Verification items for the finished model (mm, model axes). Face numbers are marked on the shaded views. Round coordinates to 2 decimals unless told otherwise and drop trailing zeros. Write each loop counter-clockwise with the first axis right and the second up, starting at its lowest first coordinate (ties: lowest second). Pieces come first, ordered by that corner, then holes. Notation, with made-up numbers: (57.5, 51) - (100.5, 51) arc R31 cw to (100.5, 82) - close; hole circle Ø9 at (75.25, 79). An arc over 180 degrees is marked (long way). Answer as a JSON object with one key per item and string values.
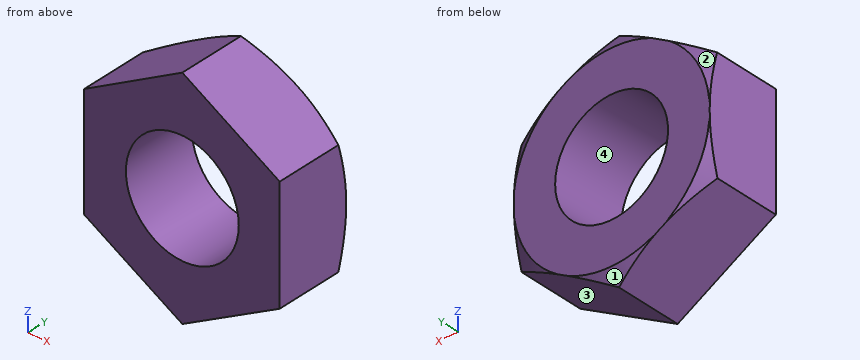
Solid Edge part; units mm, degrees
sketch "Sketch1" plane through (0, 0, 0) normal (0, -1, 0) x (1, 0, 0)
  line L0 (10.3521, 6.0691) -> (0, 12)
  line L1 (0, 12) -> (-10.4319, 5.9309)
  line L2 (-10.4319, 5.9309) -> (-10.4319, -6.0691)
  line L3 (-10.4319, -6.0691) -> (0, -12)
  line L4 (0, -12) -> (10.3521, -6.0691)
  line L5 (10.3521, -6.0691) -> (10.3521, 6.0691)
extrude "Protrusion1" add sketch "Sketch1" against normal blind 8
sketch "Sketch2" plane through (0, 0, 0) normal (0, 0, 1) x (1, 0, 0)
  line L0 (-10.4319, 8) -> (-3.0632, 12.2543)
revolve "RevolvedCutout1" cut sketch "Sketch2" angle 360 about axis through (0, 25.4232, 0) along (0, -1, 0) material side at (-6.7725, 10.1705, 0)
sketch "Sketch3" plane through (0, 0, 0) normal (0, -1, 0) x (1, 0, 0)
  circle A0 centre (0, 0) radius 6
extrude "ExtrudedCutout_1" cut sketch "Sketch3" against normal blind 10
1. Material ranges on probe 1 along X at (y, z) = (6.5, 3.25); probe 2 along Z at (x, y) = (-2.5, 4); probe 3 along Z at (x, y) = (2.75, 6.5), recorded low to high. Write a range as from..to.
Completed:
{"probe 1": "x = -10.43..-5.04, 5.04..10.35", "probe 2": "z = -10.58..-5.45, 5.45..10.55", "probe 3": "z = -10.42..-5.33, 5.33..10.42"}
2. Go/stop test with flat-tipped pins: pin 1 (1.5 mm diameter, centred on x = -3.5, z = -1.5, fed in from -Y); pin 2 (1.5 mm diameter, centred on x = 7, y = 4, fed in from -Z). Record where each tip stops, or that it passes through.
Completed:
{"pin 1": "passes through", "pin 2": "stops at z = -8.42"}
3. Cross-section at A-A (y = 5). Record the boundary of the cut face in (x, z).
Completed:
{"outline": "(-10.43, -6.07) - (0, -12) - (10.35, -6.07) - (10.35, 6.07) - (0, 12) - (-10.43, 5.93) - close; hole circle Ø12 at (0, 0)"}
4. Mould release check, pull along X, two halves, no side actions. Record for the marked faces 1, 2, 3 and 4: released by +X, released by -X, zero draft, split by the parting line, or undercut.
Completed:
{"face 1": "split by the parting line", "face 2": "released by -X", "face 3": "released by +X", "face 4": "undercut"}
